```python
from build123d import *

# Parameters (mm, degrees)
CONG_1_R       = 0.5
ECHELLE1_SCALE = 0.578571429


with BuildPart() as part:
    # Esquisse1 → Révolution1 (revolve)
    with BuildSketch(Plane.XY, mode=Mode.PRIVATE) as r_volution1_sk:
        Polygon((0, 20), (5, 20), (5, 19.25), (4.75, 19.25), (4.75, 18.75), (5, 18.75), (5, 18), (1.5, 18), (1.5, 0), (0, 0), align=None)
    revolve(r_volution1_sk.sketch.rotate(Axis((0, 0, 0), (0, 1, 0)), 90), axis=Axis((0, 0, 0), (0, 1, 0)))

    # Congé1
    cong_1_edges = [part.edges().sort_by_distance(p)[0] for p in [
        (0, 18, 1.5),
    ]]
    fillet(cong_1_edges, radius=CONG_1_R)


with BuildPart() as part_1:
    # Echelle1: scaled about (0, 14.470399807, 0)
    add(part.part.scale(ECHELLE1_SCALE).moved(Location((0, 6.098239919, 0))))


solid = part_1.part
```
Could you check a few things on this model? Use its own coordinates, in mm. A direction names the side the tool comes from. Coordinates: 2 decimals unless noted, no trailing zeros. Write each loop counter-clockwise with the first axis right and the second up, starting at its lowest first coordinate (ties: lowest second). Pieces come first, ordered by that corner, then holes. Notation, with made-up numbers: (-10.75, -13.75) -> (25.25, -13.75) arc R35 cw to (25.25, 22.25) -> close; hole circle Ø7 at (31, -31). An arc over 180 degrees is marked (long way). Write item = value, one per line. Start each with the question number.
(1) I want a section at B-B (x = 0). Please give me the cut outline in (y, z).
(2) Which directions (+Z, -Z, +X, -X, +Y, -Y) give clear straight access to the entire face, cutting with the end or side of a thin tool? Please do faces 1 (the face through (0, 17.67, 0)), 2 (the face through (1, 16.513, -1)).
(3) I want a section at A-A (z = 0). Please give me the cut outline in (x, y), plus the area to 3 significant figures.
(4) I need wall thicknesses on line 1 (Y direction, x = 1.7, z = 2.3); line 2 (Y direction, x = 1.45, z = -2); line 3 (Z direction, x = -0.7, y = 14.75). Which ranges of each line are inside material? Lowest first, please. Write a range as [from, to].
(5) Will these pins go through, and if not, where does the flat tip stop? pin 1 (1 mm diameter, centred on x = -1, y = 13.5, fed in from -Z); pin 2 (2 mm diameter, centred on x = -1, y = 10.5, fed in from -Z).
(6) I want a section at D-D (x = 2.5). Please give me the cut outline in (y, z).
(7) I want a section at C-C (y = 12). Please give me the cut outline in (x, z).
Result set:
q1.outline = (6.1, -0.87) -> (16.22, -0.87) arc R0.29 cw to (16.51, -1.16) -> (16.51, -2.89) -> (16.95, -2.89) -> (16.95, -2.75) -> (17.24, -2.75) -> (17.24, -2.89) -> (17.67, -2.89) -> (17.67, 2.89) -> (17.24, 2.89) -> (17.24, 2.75) -> (16.95, 2.75) -> (16.95, 2.89) -> (16.51, 2.89) -> (16.51, 1.16) arc R0.29 cw to (16.22, 0.87) -> (6.1, 0.87) -> close
q2.face_1 = +Z, -Z, +X, -X, +Y
q2.face_2 = -Y
q3.outline = (-2.89, 16.51) -> (-1.16, 16.51) arc R0.29 cw to (-0.87, 16.22) -> (-0.87, 6.1) -> (0.87, 6.1) -> (0.87, 16.22) arc R0.29 cw to (1.16, 16.51) -> (2.89, 16.51) -> (2.89, 16.95) -> (2.75, 16.95) -> (2.75, 17.24) -> (2.89, 17.24) -> (2.89, 17.67) -> (-2.89, 17.67) -> (-2.89, 17.24) -> (-2.75, 17.24) -> (-2.75, 16.95) -> (-2.89, 16.95) -> close
q3.area = 24.7 mm2
q4.line_1 = [16.51, 16.95], [17.24, 17.67]
q4.line_2 = [16.51, 17.67]
q4.line_3 = [-0.51, 0.51]
q5.pin_1 = -0.71
q5.pin_2 = -0.87
q6.outline = (16.51, -1.46) -> (16.95, -1.46) -> (16.95, -1.14) -> (17.24, -1.14) -> (17.24, -1.46) -> (17.67, -1.46) -> (17.67, 1.46) -> (17.24, 1.46) -> (17.24, 1.14) -> (16.95, 1.14) -> (16.95, 1.46) -> (16.51, 1.46) -> close
q7.outline = circle Ø1.74 at (0, 0)
